```python
from build123d import *

# Parameters (mm, degrees)
SKETCH_2_R               = 2.2
CUT_EXTRUDE_1_DEPTH      = 33.832910319
PATTERN_CIRCULAR_1_COUNT = 4
FILLET_1_R               = 1
CHAMFER_1_SIZE           = 1


with BuildPart() as part:
    # Эскиз1 → Повернуть1 (revolve)
    with BuildSketch(Plane.XY, mode=Mode.PRIVATE) as revolve_1_sk:
        Polygon((0, -6), (0, -11), (-2, -11), (-2, -10.75), (-4, -10.75), (-4, -21), (-8, -21), (-8, -9), (-18, -9), (-18, -6), align=None)
    revolve(revolve_1_sk.sketch.rotate(Axis((0, 0, 0), (-1, 0, 0)), 270), axis=Axis((0, 0, 0), (-1, 0, 0)))

    # Эскиз2 → Вырез-Вытянуть1 (cut, through all)
    with BuildSketch(Plane(origin=(-4, 0, 0), x_dir=(0, 0, -1), z_dir=(1, 0, 0))):
        with Locations((0, 16)):
            Circle(SKETCH_2_R)
    cut_extrude_1 = extrude(amount=-CUT_EXTRUDE_1_DEPTH, mode=Mode.SUBTRACT)

    # Круговой массив1: Вырез-Вытянуть1 ×4 about axis
    pattern_circular_1_axis = Axis((0, 0, 0), (1, 0, 0))
    for i in range(1, PATTERN_CIRCULAR_1_COUNT):
        add(cut_extrude_1.rotate(pattern_circular_1_axis, i * 360 / PATTERN_CIRCULAR_1_COUNT), mode=Mode.SUBTRACT)

    # Скругление1
    fillet_1_edges = [part.edges().sort_by_distance(p)[0] for p in [
        (-8, 0, 9),
    ]]
    fillet(fillet_1_edges, radius=FILLET_1_R)

    # Фаска1
    chamfer_1_edges = [part.edges().sort_by_distance(p)[0] for p in [
        (0, 0, 11),
        (-18, 0, 9),
    ]]
    chamfer(chamfer_1_edges, length=CHAMFER_1_SIZE)


solid = part.part
```
Here's how the part is built. I have some questions about the finished solid (model axes, mm). A direction names the side the tool comes from. Give positions to 0.01 mm unless a question says otherwise; leave off trailing zeros. Write each loop counter-clockwise with the first axis right and the second up, starting at its lowest first coordinate (ties: lowest second). Pieces come first, ordered by that corner, then holes. Notation, with made-up numbers: M 39,79 L 53,79 A26 cw 53,100 Z; hole C 13,34 d11. An arc over 180 degrees is marked long. Put each result on its own line as item: value. Start each with the question number.
Item 1: Thinking about a two-plate mould opening in Y: for faces 1 (the cylindrical face through (-6.03, -6.31, -20.03)), 2 (the cylindrical face through (-5.972, -0.477, 13.852)), 3 (the flat face through (-18, -6, 2)), 4 (the cylindrical face through (-5.972, 0.477, -13.852)), which applies, +Y half, -Y half, draft (parallel to the pull), parting line (faces both ways), or undercut?
Item 2: On a 3-axis mill with a long thin cutter (end or side, diameter ignored), from which of +Z, -Z, +X, -X, +Y, -Y can I reach the whole of each face in a straight line? I mean faces 5 (the cylindrical face through (-3.01, -7.27, 7.92)), 6 (the cylindrical face through (-1.51, 10.74, 2.38)), 7 (the flat face through (0, 7, 0)), 8 (the flat face through (-8, -5, -9)), 9 (the cylindrical face through (-5.972, -13.852, -0.477)). Say none if no direction works.
Item 3: I need wall thicknesses on L1, parallel to Y at x = -5.1, z = 0; L2, parallel to Y at x = -14, z = 0; L3, parallel to X at y = 7.5, z = -15.5. Which ranges of each line are inside material? Lowest first, please. Write a range as from..to.
Item 4: If we section it at C-C, the plane x = -4.5: Write out the boundary of the cut face in (y, z), then the cut area to 3 significant figures.
Item 5: If we section it at A-A, the plane z = 0: Count the separate pieces of the cut face and the enclosed holes in it, then the cut area to 3 significant figures.
Item 6: Will these pins go through, and if not, where does the flat tip stop? pin 1 (12 mm diameter, centred on y = -1, z = 14, fed in from -X); pin 2 (1.5 mm diameter, centred on x = -12, y = -4, fed in from +Z); pin 3 (10 mm diameter, centred on x = -6.5, z = 0.5, fed in from +Y); pin 4 (4 mm diameter, centred on y = -16, z = 0, fed in from +X).
Item 7: If we section it at D-D, the plane y = 14.5: Write out the boundary of the cut face in (x, z), then the cut area to 3 significant figures.
Values:
1. face 1: parting line
1. face 2: undercut
1. face 3: draft
1. face 4: undercut
2. face 5: none
2. face 6: +X
2. face 7: +Z, -Z, +X, +Y, -Y
2. face 8: -X
2. face 9: +X, -X
3. L1: -21..-18.2, -13.8..-6, 6..13.8, 18.2..21
3. L2: -9..-6, 6..9
3. L3: -8..-4
4. outline: C 0,0 d42; hole C -16,0 d4.4; hole C 0,0 d12; hole C 0,-16 d4.4; hole C 0,16 d4.4; hole C 16,0 d4.4
4. area: 1,210 mm²
5. separate pieces: 4
5. enclosed holes: 0
5. area: 182 mm²
6. pin 1: x = -17.96
6. pin 2: z = 8.39
6. pin 3: y = 21
6. pin 4: through
7. outline: M -8,-15.19 L -4,-15.19 L -4,-1.61 L -8,-1.61 Z; M -8,1.61 L -4,1.61 L -4,15.19 L -8,15.19 Z
7. area: 109 mm²
